Input: dimensioned drawing with shaded views. Units: mm. Origin: part minimum x, y, z. Coordinates: 2 decimals unless noted, no trailing zeros. Order: outer loops, then holes, each group sorted by start corner. A loop starts at its lowest first (then second) coordinate and runs counter-clockwise, first axis right, second up. Notation, with made-up numbers: (51, -13.75) - (69, -13.75) arc R6 ccw to (69, -9.75) - close; hole circle Ø4 at (-27, 46). An arc over 180 degrees is marked (long way). One line per question, with ' | ' between items. Start each with the question number.
(1) Section B-B (z = 3). Return the cut outline in (x, y).
(2) Draft query along X for the marked faces 1, 2, 3 and 4. Return one class per face: +X half, -X half, draft (parallel to the pull), parting line (faces both ways), or undercut.
(3) Section A-A (x = 25.4). Return the cut outline in (y, z).
(4) Contact query for flat-ended pins moving along their axis: P1, Ø10, axis at x = 39.5, z = 5.5, coming from the +Y side; P2, Ø12, axis at x = 19.5, z = 6.5, coming from the +Y side; P3, Ø20.5, axis at x = 25.4, y = 76.2, coming from the +Z side. Output: stop coordinate, or through.
(5) Section D-D (x = 5.5). Return the cut outline in (y, z).
(6) Section C-C (x = 44.5). Return the cut outline in (y, z).
(7) Line query: line 1 along Y through (x, z) = (25.4, 19); line 2 along Y through (x, z) = (31.5, 23.25); line 3 along Y through (x, z) = (46, 9). Output: solid intervals per line, ascending.
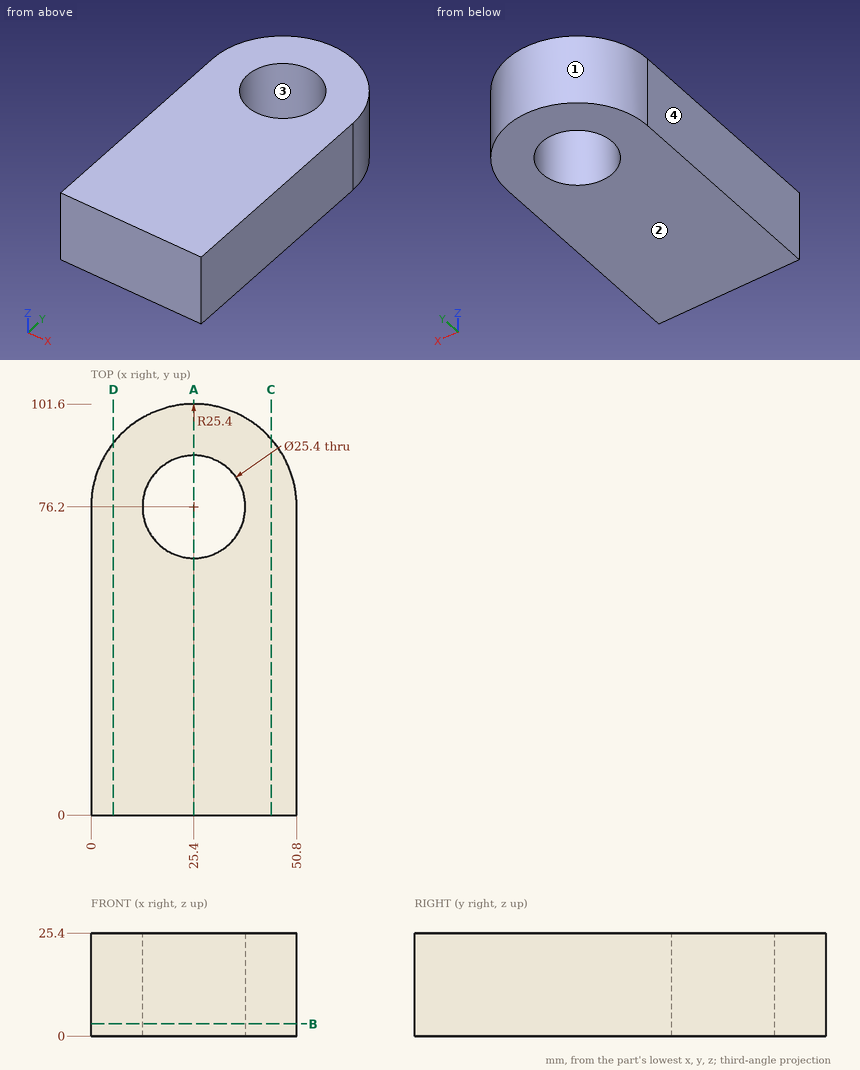
Response values:
1) outline: (0, 0) - (50.8, 0) - (50.8, 76.2) arc R25.4 ccw to (0, 76.2) - close; hole circle Ø25.4 at (25.4, 76.2)
2) face 1: parting line | face 2: draft | face 3: undercut | face 4: -X half
3) outline: (0, 0) - (63.5, 0) - (63.5, 25.4) - (0, 25.4) - close; (88.9, 0) - (101.6, 0) - (101.6, 25.4) - (88.9, 25.4) - close
4) P1: stops at y = 99.91 | P2: stops at y = 101.6 | P3: passes through
5) outline: (0, 0) - (91.98, 0) - (91.98, 25.4) - (0, 25.4) - close
6) outline: (0, 0) - (92.94, 0) - (92.94, 25.4) - (0, 25.4) - close
7) line 1: y = 0 to 63.5, 88.9 to 101.6 | line 2: y = 0 to 65.06, 87.34 to 100.86 | line 3: y = 0 to 91.06
